Read the model definition and answer for the solid it produces. Units are mm, in the model's axes. Coordinates: 2 decimals unless noted, no trailing zeros. Loops run counter-clockwise (first coordinate to the right, second up) from the corner with the lowest first, then second, coordinate; pieces in that order, holes last. Notation, with made-up numbers: (59.5, 50) -> (117.5, 50) arc R10 ccw to (117.5, 64) -> close; hole circle Ø7 at (-13, 63). An arc over 180 degrees is marked (long way). Answer as a JSON object with one key per item and string values. Group by question number.
1) Flat-ended cylindrical pins translate along their axes: P1, Ø3, axis at x = 5, y = -26, coming from the +Z side; P2, Ø2, axis at x = 29.5, y = -92, coming from the +Z side; P3, Ø4, axis at x = 23.5, y = -62.5, coming from the +Z side; P4, Ø14, axis at x = 19.05, z = 25.4, coming from the +Y side. Find the tip coordinate at first contact, or state that the pin passes through.
2) Section A-A, the plane z = 25.4 is taken. Give the vertices of the cut face in (x, y).
3) Determine the mould class of faces 1 (the face through (18.75, -75.13, 50.8)), 2 (the face through (19, -75, 0)), 3 (the face through (14.95, -75.13, 17.51)) for opening direction Z: released by +Z, released by -Z, zero draft, split by the parting line, or undercut.
4) Section C-C, the plane y = -116.5 is taken. Give the vertices of the cut face in (x, z).
5) Consider probe 1 along Z at (x, y) = (19.05, -43.5); probe 2 along X at (y, z) = (-31, 25); probe 3 along Z at (x, y) = (21.5, -130.5). Determine where each line is inside the solid, lowest interval first. Write a range as [from, to].
6) Section D-D, the plane x = 4 is taken. Give the vertices of the cut face in (y, z), plus the area to 3 significant figures.
7) Section B-B, the plane x = 19.05 is taken. Give the vertices of the cut face in (y, z), plus the area to 3 significant figures.
from build123d import *

# Parameters (mm, degrees)
F0_W     = 38.1
F0_H     = 50.8
F1_DEPTH = 152.4
F2_R     = 8.89
F3_DEPTH = 152.401
F5_W     = 152.4
F5_H     = 28.410043


with BuildPart() as f1:
    # F0 (on Front) → F1 (new body)
    with BuildSketch(Plane.XZ):
        with Locations((19.05, 25.4)):
            Rectangle(F0_W, F0_H)
    extrude(amount=F1_DEPTH)

    # F2 (on face) → F3 (cut, through all)
    with BuildSketch(Plane(origin=(0, 0, 0), x_dir=(-1, 0, 0), z_dir=(0, 1, 0))):
        with Locations((-19.05, 25.4)):
            Circle(F2_R)
    extrude(amount=-F3_DEPTH, mode=Mode.SUBTRACT)

    # F5 (on offset) → F6 (revolve, cut)
    with BuildSketch(Plane.YZ.offset(19.05)):
        with Locations((-76.2, 65.005021)):
            Rectangle(F5_W, F5_H)
    revolve(axis=Axis((19.05, -76.2, 25.4), (0, 1, 0)), mode=Mode.SUBTRACT)


solid = f1.part
Determined:
{
 "1": {"P1": "z = 47.48", "P2": "z = 48.98", "P3": "z = 50.68", "P4": "through"},
 "2": {"outline": "(0, -152.4) -> (10.16, -152.4) -> (10.16, 0) -> (0, 0) -> close; (27.94, -152.4) -> (38.1, -152.4) -> (38.1, 0) -> (27.94, 0) -> close"},
 "3": {"face 1": "released by +Z", "face 2": "released by -Z", "face 3": "undercut"},
 "4": {"outline": "(0, 8.6) arc R25.4 ccw to (38.1, 8.6) -> (38.1, 42.2) arc R25.4 ccw to (0, 42.2) -> close; hole circle Ø17.78 at (19.05, 25.4)"},
 "5": {"probe 1": "[0, 16.51], [34.29, 50.8]", "probe 2": "[0, 10.17], [27.93, 38.1]", "probe 3": "[0.12, 16.85], [33.95, 50.68]"},
 "6": {"outline": "(-152.4, 4.94) -> (0, 4.94) -> (0, 45.86) -> (-152.4, 45.86) -> close", "area": "6,240 mm²"},
 "7": {"outline": "(-152.4, 0) -> (0, 0) -> (0, 16.51) -> (-152.4, 16.51) -> close; (-152.4, 34.29) -> (0, 34.29) -> (0, 50.8) -> (-152.4, 50.8) -> close", "area": "5,030 mm²"}
}
